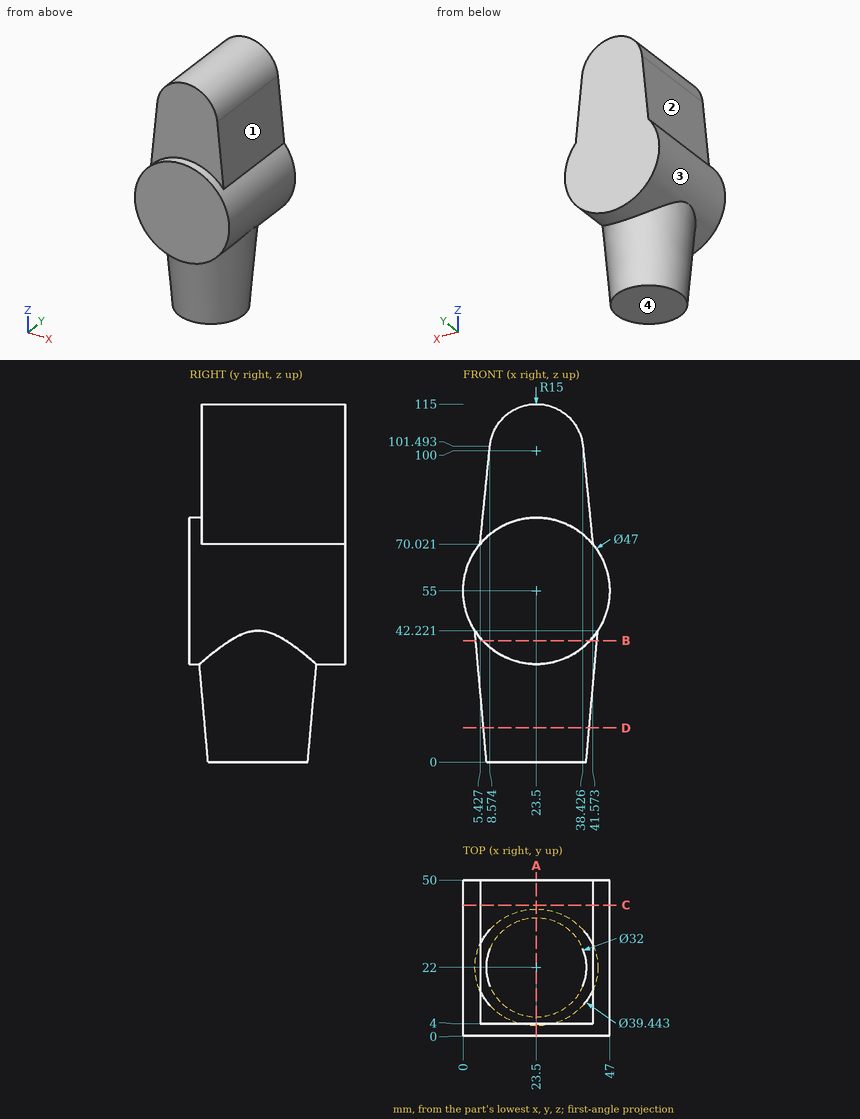
The drawing under review shows one solid part. Ordinate dimensions are in mm from its lowest x, y, z. Round coordinates to 2 decimals unless told otherwise and drop trailing zeros. Order: outer loops, then holes, each group sorted by start corner. A loop starts at its lowest first (then second) coordinate and runs counter-clockwise, first axis right, second up. Notation, with made-up numbers: (-10.5, 34) - (36.5, 34) arc R16 cw to (36.5, 63) - close; hole circle Ø6 at (-4, 38.5). An arc over 180 degrees is marked (long way). Return JSON: item names as keys, results as strings.
Q1. Consider section C-C on y = 42. Write out the cut boundary in (x, z) (1 decimal), plus the area to 3 significant figures.
Computed values:
{"outline": "(5.4, 70) arc R23.5 ccw (long way) to (41.6, 70) - (38.4, 101.5) arc R15 ccw to (8.6, 101.5) - close", "area": "2,870 mm2"}
Q2. Consider section B-B on z = 39. Write out the cut boundary in (x, y) (1 decimal), plus the area to 3 significant figures.
Computed values:
{"outline": "(6.3, 0) - (40.7, 0) - (40.7, 13) arc R19.4 ccw to (40.7, 31) - (40.7, 50) - (6.3, 50) - (6.3, 31) arc R19.4 ccw to (6.3, 13) - close", "area": "1,780 mm2"}
Q3. The part is to be moulded in two halves that separate along X. For the marked faces 1, 2, 3 and 4, say which applies: pulls with the +X half, pulls with the -X half, needs draft (parallel to the pull), parting line crosses it, or undercut.
Computed values:
{"face 1": "pulls with the +X half", "face 2": "pulls with the -X half", "face 3": "parting line crosses it", "face 4": "needs draft"}
Q4. Consider section A-A on x = 23.5. Write out the cut boundary in (y, z), plus the area to 3 significant figures.
Computed values:
{"outline": "(0, 31.5) - (3.22, 31.5) - (6, 0) - (38, 0) - (40.78, 31.5) - (50, 31.5) - (50, 115) - (4, 115) - (4, 78.5) - (0, 78.5) - close", "area": "5,120 mm2"}
Q5. Wall thickness on L1, parallel to Y at x = 9, z = 92.5; L2, parallel to X at y = 35, z = 19 (1 decimal); L3, parallel to X at y = 12, z = 24 (1 decimal): over which ranges is each line inside the solid? List them lowest first. Write a range as [from, to].
Computed values:
{"L1": "y = [4, 50]", "L2": "x = [11.5, 35.5]", "L3": "x = [8.4, 38.6]"}
Q6. Consider section D-D on z = 11. Write out the cut boundary in (x, y), plus the area to 3 significant figures.
Computed values:
{"outline": "circle Ø33.94 at (23.5, 22)", "area": "905 mm2"}
Q7. For pin 1 Ø1.5 at (y, z) = (15, 61) entering from -X; pin 2 Ø2 at (y, z) = (38.5, 37) entering from +X (1 decimal); pin 3 Ø5 at (x, y) = (18.5, 13.5) entering from +Z, all flat-tipped, find the tip position at first contact; note any pin that passes through.
Computed values:
{"pin 1": "stops at x = 0.59", "pin 2": "stops at x = 39.7", "pin 3": "stops at z = 114.79"}
